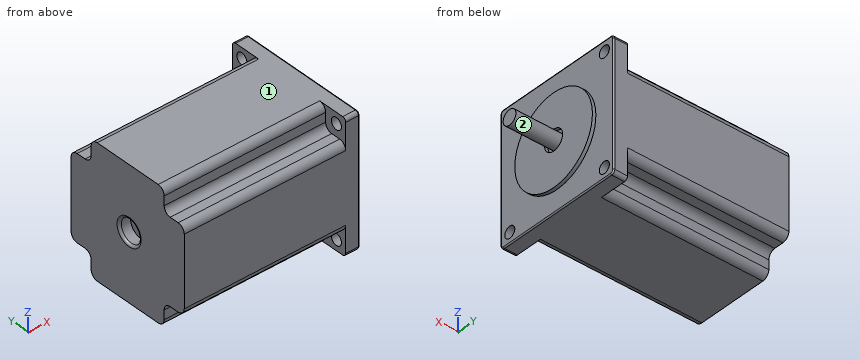
from build123d import *

# Parameters (mm, degrees)
SKETCH1_W           = 76
SKETCH1_H           = 56.4
BOSS_EXTRUDE1_DEPTH = 56.4
SKETCH2_W           = 70
SKETCH2_H           = 10
CUT_EXTRUDE1_DEPTH  = 10
SKETCH3_W           = 70
SKETCH3_H           = 10
CUT_EXTRUDE4_DEPTH  = 10
SKETCH5_W           = 70
SKETCH5_H           = 10
CUT_EXTRUDE5_DEPTH  = 10
FILLET2_R           = 3
FILLET3_R           = 3
SKETCH7_R           = 5
CUT_EXTRUDE6_DEPTH  = 5
FILLET4_R           = 1
FILLET5_R           = 0.5
FILLET6_R           = 1.5
FILLET7_R           = 1.5
SKETCH18_R          = 2.5
CUT_EXTRUDE7_DEPTH  = 10
SKETCH20_R          = 3.175
BOSS_EXTRUDE2_DEPTH = 20.6
SKETCH21_R          = 19.348505468
SKETCH21_R_2        = 4.468295999
BOSS_EXTRUDE3_DEPTH = 1.5


with BuildPart() as part:
    # Sketch1 → Boss-Extrude1 (new body)
    with BuildSketch(Plane(origin=(0, 0, 0), x_dir=(1, 0, 0), z_dir=(0, 1, 0))):
        with Locations((-12.257828935, -10.875461997)):
            Rectangle(SKETCH1_W, SKETCH1_H)
    extrude(amount=BOSS_EXTRUDE1_DEPTH)

    # Sketch2 → Cut-Extrude1 (cut)
    with BuildSketch(Plane.XY.offset(39.075461997)):
        with Locations((-15.257828935, 51.4)):
            Rectangle(SKETCH2_W, SKETCH2_H)
    extrude(amount=-CUT_EXTRUDE1_DEPTH, mode=Mode.SUBTRACT)

    # Sketch3 → Cut-Extrude4 (cut)
    with BuildSketch(Plane(origin=(0, 0, -17.324538003), x_dir=(-1, 0, 0), z_dir=(0, 0, -1))):
        with Locations((15.257828935, 51.4)):
            Rectangle(SKETCH3_W, SKETCH3_H)
        with Locations((15.257828935, 5)):
            Rectangle(SKETCH3_W, SKETCH3_H)
    extrude(amount=-CUT_EXTRUDE4_DEPTH, mode=Mode.SUBTRACT)

    # Sketch5 → Cut-Extrude5 (cut)
    with BuildSketch(Plane.XZ):
        with Locations((-15.257828935, 34.075461997)):
            Rectangle(SKETCH5_W, SKETCH5_H)
    extrude(amount=-CUT_EXTRUDE5_DEPTH, mode=Mode.SUBTRACT)

    # Fillet2
    fillet2_edges = [part.edges().sort_by_distance(p)[0] for p in [
        (-15.257828935, 56.4, 29.075461997),
        (-15.257828935, 46.4, 39.075461997),
        (-15.257828935, 0, -7.324538003),
        (-15.257828935, 10, -17.324538003),
        (-15.257828935, 56.4, -7.324538003),
        (-15.257828935, 46.4, -17.324538003),
        (-15.257828935, 10, 39.075461997),
        (-15.257828935, 0, 29.075461997),
    ]]
    fillet(fillet2_edges, radius=FILLET2_R)

    # Fillet3
    fillet3_edges = [part.edges().sort_by_distance(p)[0] for p in [
        (-15.257828935, 46.4, 29.075461997),
        (-15.257828935, 10, -7.324538003),
        (-15.257828935, 46.4, -7.324538003),
        (-15.257828935, 10, 29.075461997),
    ]]
    fillet(fillet3_edges, radius=FILLET3_R)

    # Sketch7 → Cut-Extrude6 (cut)
    with BuildSketch(Plane.ZY.offset(50.257828935)):
        with Locations((11.575461997, 27.5)):
            Circle(SKETCH7_R)
    extrude(amount=-CUT_EXTRUDE6_DEPTH, mode=Mode.SUBTRACT)

    # Fillet4
    fillet4_edges = [part.edges().sort_by_distance(p)[0] for p in [
        (-50.257828935, 27.5, 6.575461997),
    ]]
    fillet(fillet4_edges, radius=FILLET4_R)

    # Fillet5
    fillet5_edges = [part.edges().sort_by_distance(p)[0] for p in [
        (25.742171065, 56.4, 10.875461997),
        (25.742171065, 0, 10.875461997),
        (25.742171065, 28.2, -17.324538003),
        (25.742171065, 28.2, 39.075461997),
    ]]
    fillet(fillet5_edges, radius=FILLET5_R)

    # Fillet6
    # the kernel refuses this fillet: 1.5 mm, written as the material it takes off along each edge
    with BuildSketch(Plane(origin=(25.742171065, 54.9, 37.575461997), x_dir=(0, 1, 0), z_dir=(0, 0, -1))) as fillet6_piece_1:
        with BuildLine():
            CenterArc((1, -0.5), 0.5, 0, 90)
            Line((1.5, -0.5), (1.5, 0))
            Line((1.5, 0), (1, 0))
        make_face()
    revolve(axis=Axis((25.742171065, 54.9, 37.575461997), (1, 0, 0)), revolution_arc=90, mode=Mode.SUBTRACT)
    with BuildSketch(Plane(origin=(25.742171065, 56.4, 39.075461997), x_dir=(0, -1, 0), z_dir=(-1, 0, 0))) as fillet6_piece_2:
        with BuildLine():
            CenterArc((FILLET6_R, -FILLET6_R), FILLET6_R, 90, 90)
            Line((0, -FILLET6_R), (0, 0))
            Line((0, 0), (FILLET6_R, 0))
        make_face()
    extrude(amount=9.75, mode=Mode.SUBTRACT)

    # Fillet7
    # the kernel refuses this fillet: 1.5 mm, written as the material it takes off along each edge
    with BuildSketch(Plane(origin=(25.742171065, 1.5, 37.575461997), x_dir=(0, 0, 1), z_dir=(0, 1, 0))) as fillet7_piece_1:
        with BuildLine():
            CenterArc((1, -0.5), 0.5, 0, 90)
            Line((1.5, -0.5), (1.5, 0))
            Line((1.5, 0), (1, 0))
        make_face()
    revolve(axis=Axis((25.742171065, 1.5, 37.575461997), (1, 0, 0)), revolution_arc=90, mode=Mode.SUBTRACT)
    with BuildSketch(Plane(origin=(25.742171065, 54.9, -15.824538003), x_dir=(0, 0, -1), z_dir=(0, -1, 0))) as fillet7_piece_2:
        with BuildLine():
            CenterArc((1, -0.5), 0.5, 0, 90)
            Line((1.5, -0.5), (1.5, 0))
            Line((1.5, 0), (1, 0))
        make_face()
    revolve(axis=Axis((25.742171065, 54.9, -15.824538003), (1, 0, 0)), revolution_arc=90, mode=Mode.SUBTRACT)
    with BuildSketch(Plane(origin=(25.742171065, 1.5, -15.824538003), x_dir=(0, -1, 0), z_dir=(0, 0, 1))) as fillet7_piece_3:
        with BuildLine():
            CenterArc((1, -0.5), 0.5, 0, 90)
            Line((1.5, -0.5), (1.5, 0))
            Line((1.5, 0), (1, 0))
        make_face()
    revolve(axis=Axis((25.742171065, 1.5, -15.824538003), (1, 0, 0)), revolution_arc=90, mode=Mode.SUBTRACT)
    with BuildSketch(Plane(origin=(15.992171065, 56.4, -17.324538003), x_dir=(0, -1, 0), z_dir=(1, 0, 0)), Plane(origin=(15.992171065, 0, -17.324538003), x_dir=(0, 0, 1), z_dir=(1, 0, 0)), Plane(origin=(25.742171065, 0, 39.075461997), x_dir=(0, 0, -1), z_dir=(-1, 0, 0))) as fillet7_piece_4:
        with BuildLine():
            CenterArc((FILLET7_R, -FILLET7_R), FILLET7_R, 90, 90)
            Line((0, -FILLET7_R), (0, 0))
            Line((0, 0), (FILLET7_R, 0))
        make_face()
    extrude(amount=9.75, mode=Mode.SUBTRACT)

    # Sketch18 → Cut-Extrude7 (cut)
    with BuildSketch(Plane(origin=(25.742171065, 0, 0), x_dir=(0, 0, -1), z_dir=(1, 0, 0))):
        with Locations((-34.445461997, 51.77)):
            Circle(SKETCH18_R)
        with Locations((12.694538003, 51.77)):
            Circle(SKETCH18_R)
        with Locations((12.694538003, 4.63)):
            Circle(SKETCH18_R)
        with Locations((-34.445461997, 4.63)):
            Circle(SKETCH18_R)
    extrude(amount=-CUT_EXTRUDE7_DEPTH, mode=Mode.SUBTRACT)

    # Sketch20 → Boss-Extrude2 (add)
    with BuildSketch(Plane(origin=(25.742171065, 0, 0), x_dir=(0, 0, -1), z_dir=(1, 0, 0))):
        with Locations(Location((-10.875461997, 28.2, 0), (0, 0, 180))):
            Circle(SKETCH20_R)
    extrude(amount=BOSS_EXTRUDE2_DEPTH)

    # Sketch21 → Boss-Extrude3 (add)
    with BuildSketch(Plane(origin=(25.742171065, 0, 0), x_dir=(0, 0, -1), z_dir=(1, 0, 0))):
        with Locations(Location((-10.875461997, 28.2, 0), (0, 0, 180))):
            Circle(SKETCH21_R)
        with Locations((-10.875461997, 28.2)):
            Circle(SKETCH21_R_2, mode=Mode.SUBTRACT)
    extrude(amount=BOSS_EXTRUDE3_DEPTH)


solid = part.part
Build history of the part. All positions in model axes, mm. Face numbers are marked on the shaded views. A direction names the side the tool comes from. Coordinates: 2 decimals unless noted, no trailing zeros. Write each loop counter-clockwise with the first axis right and the second up, starting at its lowest first coordinate (ties: lowest second). Pieces come first, ordered by that corner, then holes.
(1) 3-axis set-ups, long thin cutter, end or side, ignore diameter. For the marked faces 1 and 2: which of +Z, -Z, +X, -X, +Y, -Y reach the whole face in a straight line?
(2) Pin check, flat tips, straight feed: pin 1 Ø10.5 at (y, z) = (6, 33) entering from -X; pin 2 Ø3 at (x, y) = (-11.5, 5.5) entering from -Z; pin 3 Ø2 at (x, y) = (-13, 4) entering from +Z; pin 4 Ø2 at (x, z) = (-10, 34) entering from -Y. Stop position of each tip, or through.
(3) Cut at A-A on y = 4.63. List the corners of the cut face in (x, z), and give its area (3 significant figures).
(4) Cut at D-D on y = 39.5. List the corners of the cut face in (x, z).
(5) Cut at B-B on x = -26.5. List the corners of the cut face in (y, z).
(6) Drill centre lines: line 1 (Z direction, x = -46, y = 27); line 2 (X direction, y = 47, z = 24.5); line 3 (Y direction, x = -31.5, z = 35). Where is each one in solid material? Low to high.
(7) Cut at C-C on z = 22.5. List the corners of the cut face in (x, y).
Working result:
1. face 1: +Z, +X, -X, +Y, -Y
1. face 2: +X
2. pin 1: stops at x = -50.26
2. pin 2: stops at z = -7.32
2. pin 3: stops at z = 29.08
2. pin 4: stops at y = 10
3. outline: (-50.26, -7.32) - (19.74, -7.32) - (19.74, -10.19) - (25.74, -10.19) - (25.74, 31.95) - (19.74, 31.95) - (19.74, 29.08) - (-50.26, 29.08) - close; (19.74, -17.32) - (25.24, -17.32) arc R0.5 ccw to (25.74, -16.82) - (25.74, -15.19) - (19.74, -15.19) - close; (19.74, 36.95) - (25.74, 36.95) - (25.74, 38.58) arc R0.5 ccw to (25.24, 39.08) - (19.74, 39.08) - close
3. area: 2,830 mm2
4. outline: (-50.26, -17.32) - (25.24, -17.32) arc R0.5 ccw to (25.74, -16.82) - (25.74, -4.83) - (27.24, -4.83) - (27.24, 26.58) - (25.74, 26.58) - (25.74, 38.58) arc R0.5 ccw to (25.24, 39.08) - (-50.26, 39.08) - close
5. outline: (0, -4.32) arc R3 ccw to (3, -7.32) - (7, -7.32) arc R3 cw to (10, -10.32) - (10, -14.32) arc R3 ccw to (13, -17.32) - (43.4, -17.32) arc R3 ccw to (46.4, -14.32) - (46.4, -10.32) arc R3 cw to (49.4, -7.32) - (53.4, -7.32) arc R3 ccw to (56.4, -4.32) - (56.4, 26.08) arc R3 ccw to (53.4, 29.08) - (49.4, 29.08) arc R3 cw to (46.4, 32.08) - (46.4, 36.08) arc R3 ccw to (43.4, 39.08) - (13, 39.08) arc R3 ccw to (10, 36.08) - (10, 32.08) arc R3 cw to (7, 29.08) - (3, 29.08) arc R3 ccw to (0, 26.08) - close
6. line 1: z = -17.32 to 6.6, 16.55 to 39.08
6. line 2: x = -50.26 to 25.74
6. line 3: y = 10 to 46.4
7. outline: (-50.26, 0) - (25.24, 0) arc R0.5 ccw to (25.74, 0.5) - (25.74, 12.73) - (27.24, 12.73) - (27.24, 43.67) - (25.74, 43.67) - (25.74, 55.9) arc R0.5 ccw to (25.24, 56.4) - (-50.26, 56.4) - close
